Design review of the part shown in the three views and the two pictorial views. Dimensions are in mm from the part's minimum x, y and z. Round coordinates to 2 decimals unless told otherwise and drop trailing zeros. Order: outer loops, then holes, each group sorted by start corner. A loop starts at its lowest first (then second) coordinate and runs counter-clockwise, first axis right, second up.
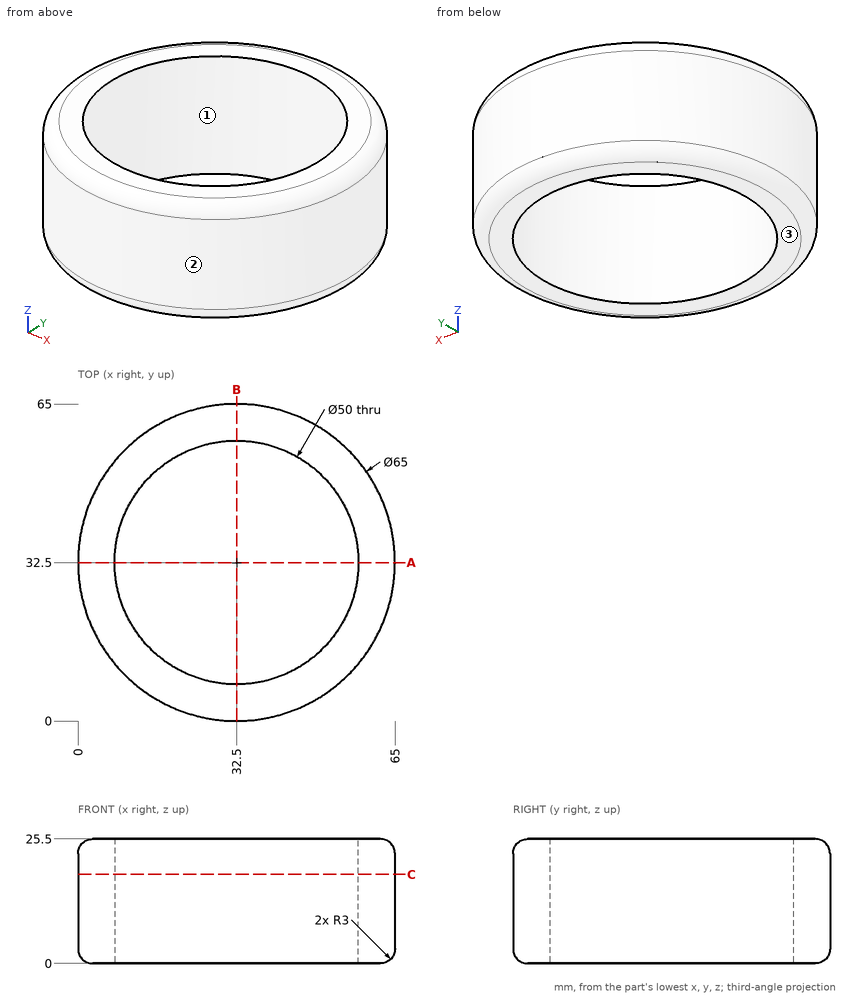
(1) Consider section C-C (z = 18.25). Write out the cut boundary in (x, y).
Data:
outline: circle Ø65 at (32.5, 32.5); hole circle Ø50 at (32.5, 32.5)
(2) To check wall thickness, follow probe 1 along Y at (x, z) = (32.5, 12); probe 2 along X at (y, z) = (38, 2); probe 3 along X at (y, z) = (25.5, 19.75). State the ranges of each line that lie inside material, in increasing order.
Data:
probe 1: y = 0 to 7.5, 57.5 to 65
probe 2: x = 0.64 to 8.11, 56.89 to 64.36
probe 3: x = 0.76 to 8.5, 56.5 to 64.24
(3) Consider section A-A (y = 32.5). Write out the cut boundary in (x, z).
Data:
outline: (0, 3) arc R3 ccw to (3, 0) - (7.5, 0) - (7.5, 25.5) - (3, 25.5) arc R3 ccw to (0, 22.5) - close; (57.5, 0) - (62, 0) arc R3 ccw to (65, 3) - (65, 22.5) arc R3 ccw to (62, 25.5) - (57.5, 25.5) - close
(4) Insertion check: pin 1 (1 mm diameter, centred on y = 14.5, z = 5.5, fed in from +X); pin 2 (3 mm diameter, centred on y = 26.5, z = 22, fed in from +X); pin 3 (6 mm diameter, centred on y = 7, z = 6.5, fed in from -X). Each pin has a flat end and moves straight along its axis. Give the tip position at first contact, or say it passes through.
Data:
pin 1: stops at x = 59.89
pin 2: stops at x = 64.69
pin 3: stops at x = 9.05
(5) Draft analysis for pull direction X (two halves, no side actions). For the marked faces 1, 2 and 3, state which applies: pulls with the +X half, pulls with the -X half, needs draft (parallel to the pull), parting line crosses it, or undercut.
Data:
face 1: undercut
face 2: parting line crosses it
face 3: needs draft
